Autodesk Inventor part; units mm, degrees
ref_plane "YZ Plane" through (0, 0, 0) normal (1, 0, 0) x (0, 1, 0)
ref_plane "XZ Plane" through (0, 0, 0) normal (0, 1, 0) x (-1, 0, 0)
ref_plane "XY Plane" through (0, 0, 0) normal (0, 0, 1) x (1, 0, 0)
sketch "Sketch1" plane through (0, 0, 0) normal (0, 0, 1) x (1, 0, 0)
  line L0 (0, 0) -> (24.5, 0)
  line L1 (24.5, 0) -> (24.5, 19.5)
  line L2 (24.5, 19.5) -> (0, 19.5)
  line L3 (0, 19.5) -> (0, 0)
  dimension "d0" = 19.5
  dimension "d1" = 24.5
extrude "Extrusion1" add sketch "Sketch1" along normal blind 36.5
sketch "Sketch12" plane through (0, 0, 0) normal (0, -1, 0) x (1, 0, 0)
  line L0 (24.5, 0) -> (24.5, 36.5)
  line L1 (0, 0) -> (0, 36.5)
  line L2 (24.5, 0) -> (24.5, 36.5)
  line L3 (24.5, 9.75) -> (24.5, 0)
  line L4 (0, 0) -> (24.5, 0)
  line L5 (14.75, 0) -> (24.5, 9.75)
  line L6 (0, 0) -> (0, 36.5)
  line L7 (0, 9.75) -> (9.75, 0)
  line L8 (9.75, 0) -> (0, 0)
  line L9 (0, 0) -> (0, 9.75)
  dimension "d75" = 5
  dimension "d76" = 45
  dimension "d77" = 45
  dimension "d79" = 9.75
extrude "Extrusion10" cut sketch "Sketch12" against normal through all
sketch "Sketch2" plane through (0, 0, 36.5) normal (0, 0, 1) x (1, 0, 0)
  line L0 (6.5, 9.5) -> (24.5, 9.5)
  line L1 (24.5, 9.5) -> (24.5, 19.5)
  line L2 (24.5, 19.5) -> (6.5, 19.5)
  line L3 (6.5, 19.5) -> (6.5, 9.5)
  line L4 (0, 0) -> (24.5, 0)
  line L5 (24.5, 0) -> (24.5, 19.5)
  line L6 (24.5, 19.5) -> (0, 19.5)
  dimension "d4" = 10
  dimension "d6" = 18
extrude "Extrusion2" add sketch "Sketch2" along normal blind 65
sketch "Sketch3" plane through (6.5, 9.5, 36.5) normal (0, -1, 0) x (1, 0, 0)
  circle A0 centre (9, 15) radius 4.95
  line L0 (18, 0) -> (18, 65)
  line L1 (18, 0) -> (0, 0)
  line L2 (0, 65) -> (18, 65)
  point P0 (-6.5, -36.5)
  point P1 (9, 65)
  dimension "d9" = 9.9
  dimension "d11" = 15
extrude "Extrusion3" cut sketch "Sketch3" against normal up to next
sketch "Sketch9" plane through (6.5, 19.5, 35) normal (0, 1, 0) x (1, 0, 0)
  circle A0 centre (9, -55) radius 4
  line L0 (18, -66.5) -> (0, -66.5)
  line L1 (18, 0) -> (0, 0)
  point P0 (-6.5, 35)
  point P1 (9, -66.5)
  dimension "d42" = 8
  dimension "d43" = 55
extrude "Extrusion9" add sketch "Sketch9" along normal blind 10
sketch "Sketch14" plane through (0, 0, 36.5) normal (0, 0, 1) x (1, 0, 0)
  line L0 (24.5, 9.5) -> (6.5, 9.5)
  line L1 (24.5, 9.5) -> (6.5, 9.5)
  line L2 (6.5, 9.5) -> (6.5, -5)
  line L3 (6.5, -5) -> (24.5, -5)
  line L4 (24.5, -5) -> (24.5, 9.5)
  line L5 (6.5, 9.5) -> (6.5, 19.5)
  line L6 (0, 0) -> (24.5, 0)
  dimension "d89" = 5
extrude "Extrusion11" add sketch "Sketch14" along normal blind 5
fillet "Fillet3" radius 9 2 edges at (24.5, 14.5, 101.5) (6.5, 14.5, 101.5)
fillet "Fillet1" radius 2 15 edges at (12.25, 0, 0) (24.5, 0, 23.125) (0, 0, 23.125) (0, 19.5, 23.125) (12.25, 19.5, 0) (21.864, 19.5, 98.864) (9.136, 19.5, 98.864) (6.5, 19.5, 64.5001) (21.864, 9.5, 98.864) (15.5, 9.5, 101.5) (24.5, 9.5, 67.0001) (6.5, 9.5, 67.0001) (24.5, 2.25, 41.5) (24.5, -5, 39) (15.5, -5, 41.5)
fillet "Fillet5" radius 0.5 2 edges at (10.55, 9.5, 51.5) (10.55, 19.5, 51.5)
fillet "Fillet6" radius 0.5 1 edges at (11.5, 29.5, 90)
sketch "Sketch10" plane through (15.5, 29.5, 90) normal (0, 1, 0) x (1, 0, 0)
  point P0 (-15.5, 90)
  point P1 (0, 0)
hole "Upper Arm Cap Hole" at (15.5, 29.5, 90) direction (0, -1, 0) diameter 3 depth 8 tip angle 118 countersink diameter 4 countersink angle 90
sketch "Sketch13" plane through (0, 0, 0) normal (0, 0, -1) x (-1, 0, 0)
  line L0 (-14.75, 17.5) -> (-14.75, 2)
  line L1 (-9.75, 2) -> (-14.75, 2)
  point P0 (0, 0)
  point P1 (-12.25, 9.75)
  point P2 (-14.75, 9.75)
  point P3 (-12.25, 2)
hole "Hole3" at (12.25, 9.75, 0) direction (0, 0, 1) diameter 3 depth 10 tip angle 118 countersink diameter 4 countersink angle 90
properties part number "Lift Mount Right"
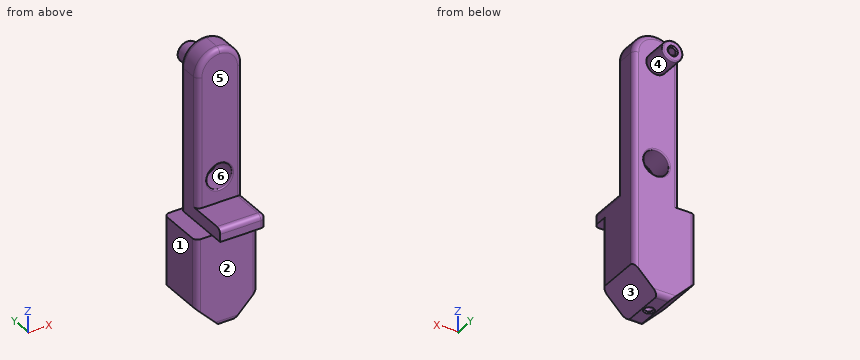
Verification items for the finished model (mm, model axes). Face numbers are marked on the shaded views. A direction names the side the tool comes from. Round coordinates to 2 decimals unless told otherwise and drop trailing zeros. Write each loop counter-clockwise with the first axis right and the second up, starting at its lowest first coordinate (ties: lowest second). Pieces come first, ordered by that corner, then holes.
1. Draft check along Z on the marked faces 3, 4, 5 and 6. Enter one of: +Z half, -Z half, draft (parallel to the pull), parting line (faces both ways), or undercut.
2. Section check A-A on z = 51.5. Enter the section's corners in (x, y), plus the area to 3 significant figures.
3. Section check D-D on y = 3. Enter the section's corners in (x, z), plus the area to 3 significant figures.
4. Section check B-B on y = -1. Enter the section's corners in (x, z).
5. Section check C-C on z = 31. Enter the section's corners in (x, y), plus the area to 3 significant figures.
6. Scan lines: L1, parallel to X at y = 23.5, z = 90; L2, parallel to Y at x = 20.25, z = 76; L3, parallel to Y at x = 12, z = 14.5. Record each from-to range of solid material in increasing order.
7. Gauge pin test, flat ends, axial feed: P1, Ø2.5, axis at x = 15.5, z = 90, coming from the -Y side; P2, Ø3, axis at x = 4, y = -1, coming from the +Z side; P3, Ø4.5, axis at x = 11.5, y = 4, coming from the +Z side; P4, Ø5, axis at x = 12.25, y = 9.75, coming from the -Z side. Record the tip position at first contact, or that the pin passes through.
8. Access from +Z, -Z, +X, -X, +Y, -Y to the whole of each face (thin tool, end or side, straight path). Record for the marked faces 1 and 2.
Answer:
1. face 3: -Z half
1. face 4: parting line
1. face 5: draft
1. face 6: undercut
2. outline: (6.5, 11.5) arc R2 ccw to (8.5, 9.5) - (10.05, 9.5) arc R0.5 ccw to (10.55, 10) - (10.55, 19) arc R0.5 ccw to (10.05, 19.5) - (8.5, 19.5) arc R2 ccw to (6.5, 17.5) - close; (20.45, 10) arc R0.5 ccw to (20.95, 9.5) - (22.5, 9.5) arc R2 ccw to (24.5, 11.5) - (24.5, 17.5) arc R2 ccw to (22.5, 19.5) - (20.95, 19.5) arc R0.5 ccw to (20.45, 19) - close
2. area: 77.4 mm2
3. outline: (0, 9.75) - (9.75, 0) - (14.75, 0) - (24.5, 9.75) - (24.5, 39.5) arc R2 ccw to (22.5, 41.5) - (6.5, 41.5) - (6.5, 36.5) - (0, 36.5) - close
3. area: 888 mm2
4. outline: (6.5, 36.5) - (24.5, 36.5) - (24.5, 39.5) arc R2 ccw to (22.5, 41.5) - (6.5, 41.5) - close
5. outline: (0, 2) arc R2 ccw to (2, 0) - (22.5, 0) arc R2 ccw to (24.5, 2) - (24.5, 17.5) arc R2 ccw to (22.5, 19.5) - (2, 19.5) arc R2 ccw to (0, 17.5) - close
5. area: 474 mm2
6. L1: x = 11.5 to 14, 17 to 19.5
6. L2: y = 9.5 to 19.5
6. L3: y = 0 to 19.5
7. P1: stops at y = 9.5
7. P2: stops at z = 36.5
7. P3: stops at z = 41.5
7. P4: stops at z = 0
8. face 1: +Z, -Z, -X, +Y, -Y
8. face 2: -Z, +X, -X, -Y
